```python
from build123d import *

# Parameters (mm, degrees)
F1_DEPTH  = 3.175
F2_R      = 4.6355
F3_DEPTH  = 15.875
F4_SIZE   = 1.5875
F6_R      = 6.35
F7_DEPTH  = 17.145
F9_DEPTH  = 6.35
F11_DEPTH = 6.35


with BuildPart() as f1:
    # F0 (on Front) → F1 (new body, symmetric)
    with BuildSketch(Plane.XZ):
        with BuildLine():
            Line((0, 179.4002), (0, 0))
            Line((0, 0), (377.5202, 0))
            Line((377.5202, 0), (428.4760097452, 58.1765707746))
            ThreePointArc((428.4760097452, 58.1765707746), (432.588720587, 75.4986793815), (420.5927391638, 88.6541446621))
            Line((420.5927391638, 88.6541446621), (168.275, 179.4002))
            Line((168.275, 179.4002), (0, 179.4002))
        make_face()
    extrude(amount=F1_DEPTH, both=True)

    # F2 (on face) → F3 (join)
    with BuildSketch(Plane.XZ.offset(3.175)):
        with Locations((23.622, 70.7136)):
            Circle(F2_R)
        with Locations((98.2218, 54.8386)):
            Circle(F2_R)
        with Locations((339.5218, 54.8386)):
            Circle(F2_R)
        with Locations((136.7282, 95.3262)):
            Circle(F2_R)
        with Locations((47.8282, 154.051)):
            Circle(F2_R)
        with Locations((117.6782, 123.9012)):
            Circle(F2_R)
        with Locations((414.147, 70.7136)):
            Circle(F2_R)
    extrude(amount=F3_DEPTH)

    # F4
    f4_edges = [f1.edges().sort_by_distance(p)[0] for p in [
        (18.9865, -19.05, 70.7136),
        (43.1927, -19.05, 154.051),
        (93.5863, -19.05, 54.8386),
        (113.0427, -19.05, 123.9012),
        (132.0927, -19.05, 95.3262),
        (334.8863, -19.05, 54.8386),
        (409.5115, -19.05, 70.7136),
    ]]
    chamfer(f4_edges, length=F4_SIZE)

    # F6 (on face) → F7 (join)
    with BuildSketch(Plane.XZ.offset(3.175)):
        with Locations((385.572, 70.7136)):
            Circle(F6_R)
        with Locations((52.197, 70.7136)):
            Circle(F6_R)
    extrude(amount=F7_DEPTH)

    # F8 (on face) → F9 (join)
    with BuildSketch(Plane.XZ.offset(20.32)):
        with BuildLine():
            ThreePointArc((58.9407, 77.0636), (52.197, 83.8073), (45.4533, 77.0636))
            Line((45.4533, 77.0636), (45.4533, 64.3636))
            ThreePointArc((45.4533, 64.3636), (52.197, 57.6199), (58.9407, 64.3636))
            Line((58.9407, 64.3636), (58.9407, 77.0636))
        make_face()
    extrude(amount=F9_DEPTH)

    # F10 (on face) → F11 (join)
    with BuildSketch(Plane.XZ.offset(20.32)):
        with BuildLine():
            ThreePointArc((387.8424602375, 70.7136), (391.0851112991, 73.1799041451), (392.3157, 77.0636))
            ThreePointArc((392.3157, 77.0636), (385.572, 83.8073), (378.8283, 77.0636))
            ThreePointArc((378.8283, 77.0636), (380.0588887009, 73.1799041451), (383.3015397625, 70.7136))
            ThreePointArc((383.3015397625, 70.7136), (385.572, 71.1073), (387.8424602375, 70.7136))
        make_face()
        with BuildLine():
            Line((392.3157, 64.3636), (392.3157, 77.0636))
            ThreePointArc((392.3157, 77.0636), (391.0851112991, 73.1799041451), (387.8424602375, 70.7136))
            ThreePointArc((387.8424602375, 70.7136), (391.0851112991, 68.2472958549), (392.3157, 64.3636))
        make_face()
        with BuildLine():
            ThreePointArc((383.3015397625, 70.7136), (380.0588887009, 73.1799041451), (378.8283, 77.0636))
            Line((378.8283, 77.0636), (378.8283, 64.3636))
            ThreePointArc((378.8283, 64.3636), (380.0588887009, 68.2472958549), (383.3015397625, 70.7136))
        make_face()
        with BuildLine():
            ThreePointArc((392.3157, 64.3636), (391.0851112991, 68.2472958549), (387.8424602375, 70.7136))
            ThreePointArc((387.8424602375, 70.7136), (385.572, 70.3199), (383.3015397625, 70.7136))
            ThreePointArc((383.3015397625, 70.7136), (380.0588887009, 68.2472958549), (378.8283, 64.3636))
            ThreePointArc((378.8283, 64.3636), (385.572, 57.6199), (392.3157, 64.3636))
        make_face()
        with BuildLine():
            ThreePointArc((383.3015397625, 70.7136), (385.572, 70.3199), (387.8424602375, 70.7136))
            ThreePointArc((387.8424602375, 70.7136), (385.572, 71.1073), (383.3015397625, 70.7136))
        make_face()
    extrude(amount=F11_DEPTH)


solid = f1.part
```
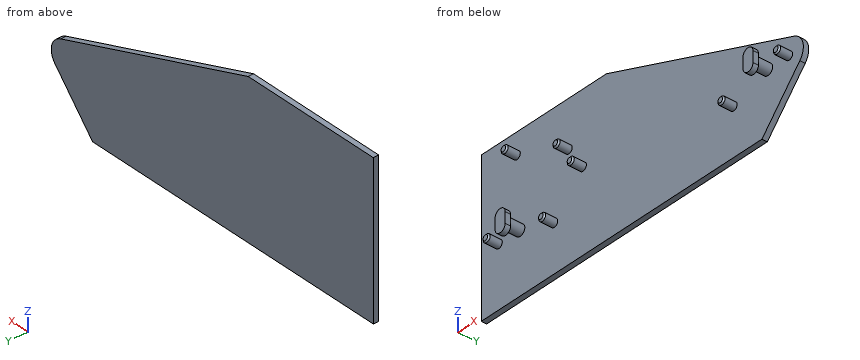
The listing builds one solid part. Answer for the finished solid, in the listing's coordinates (mm). Round coordinates to 2 decimals unless told otherwise and drop trailing zeros. Write each loop counter-clockwise with the first axis right and the second up, starting at its lowest first coordinate (ties: lowest second). Pieces come first, ordered by that corner, then holes. Notation, with made-up numbers: (-27.5, 70.25) -> (16.5, 70.25) arc R18 cw to (16.5, 77.25) -> close; hole circle Ø7 at (42, 16). An arc over 180 degrees is marked (long way). Answer as a JSON object with one key per item and string values. Group by question number.
Q1. Section A-A (y = -12.75) is taken. Count the separate pieces of the cut face and the enclosed holes in it, plus the area to 3 significant figures.
Q2. Section B-B (x = 160) is taken. Write down the section's boundary in (y, z) (3 decimals), plus the area to 3 significant figures.
Q3. Section C-C (z = 133.5) is taken. Write down the section's boundary in (x, y) (3 decimals), plus the area to 3 significant figures.
Q4. Each of these flat-tipped pins is pushed along its axis until it touches: pin 1 Ø6 at (y, z) = (-14.5, 122.5) entering from +X; pin 2 Ø5 at (y, z) = (-23.5, 71) entering from +X; pin 3 Ø6 at (y, z) = (-20.5, 56) entering from +X. Where does it stop, or does it pass through?
Q5. Straight lines are drawn through the part: line 1 along Y through (x, z) = (20.5, 41.5) (3 decimals); line 2 along Z through (x, y) = (118.5, -12); line 3 along X through (y, z) = (-6.75, 52.5). For each, find the intervals that lie inside material, in ascending order.
Check values:
{
 "1": {"separate pieces": "9", "enclosed holes": "0", "area": "726 mm^2"},
 "2": {"outline": "(-3.175, 0) -> (3.175, 0) -> (3.175, 179.4) -> (-3.175, 179.4) -> close", "area": "1,140 mm^2"},
 "3": {"outline": "(0, -3.175) -> (295.9, -3.175) -> (295.9, 3.175) -> (0, 3.175) -> close", "area": "1,880 mm^2"},
 "4": {"pin 1": "x = 122.31", "pin 2": "x = 392.32", "pin 3": "x = 389.66"},
 "5": {"line 1": "-3.175 to 3.175", "line 2": "119.34 to 128.46", "line 3": "94.22 to 102.22, 335.52 to 343.52"}
}
